Read the model definition and answer for the solid it produces. Units are mm, in the model's axes. A direction names the side the tool comes from. Coordinates: 2 decimals unless noted, no trailing zeros. Loops run counter-clockwise (first coordinate to the right, second up) from the corner with the lowest first, then second, coordinate; pieces in that order, holes last. Notation, with made-up numbers: (-2.5, 24) - (47.5, 24) arc R36 ccw to (47.5, 60) - close; hole circle Ø1 at (-9.5, 36.25). An arc over 180 degrees is marked (long way). One line per item, written item: value. Start each with the question number.
from build123d import *
from build123d.topology import SkipClean

# Parameters (mm, degrees)
SKETCH_1_R               = 27.5
EXTRUDE_1_DEPTH          = 4.5
SKETCH_2_R               = 9.75
EXTRUDE_2_DEPTH          = 30.8
CUT_EXTRUDE_1_DEPTH      = 28
SKETCH_5_R               = 10
EXTRUDE_3_DEPTH          = 7
SKETCH_6_R               = 8.5
EXTRUDE_4_DEPTH          = 8
SKETCH_11_R              = 2.5
CUT_EXTRUDE_3_DEPTH      = 50.609878049
PATTERN_CIRCULAR_1_COUNT = 6
SKETCH_12_R              = 13.008113322
CUT_EXTRUDE_4_DEPTH      = 25.8
CHAMFER_2_SIZE           = 1
SKETCH_13_W              = 0.4
SKETCH_13_H              = 1.1
CHAMFER_3_SIZE           = 0.5
CUT_EXTRUDE_5_DEPTH      = 46.964660338
SKETCH_15_R              = 1.6
CUT_EXTRUDE_6_DEPTH      = 25
HOLE_WIZARD_M3_1_D       = 2.5
SKETCH_18_R              = 27.5
CUT_EXTRUDE_7_DEPTH      = 44.505746792
PATTERN_CIRCULAR_2_COUNT = 3
PATTERN_CIRCULAR_2_ANGLE = 240
SKETCH_19_R              = 5
CUT_EXTRUDE_8_DEPTH      = 1


with BuildPart() as part:
    # 草图1 → 凸台-拉伸1 (new body)
    with BuildSketch(Plane(origin=(0, 0, 0), x_dir=(1, 0, 0), z_dir=(0, 1, 0))):
        with Locations(Location((0, 0, 0), (0, 0, 270))):
            Circle(SKETCH_1_R)
    extrude(amount=EXTRUDE_1_DEPTH)

    # 草图2 → 凸台-拉伸2 (add)
    with BuildSketch(Plane(origin=(0, 4.5, 0), x_dir=(1, 0, 0), z_dir=(0, 1, 0))):
        with Locations(Location((0, 0, 0), (0, 0, 90))):
            Circle(SKETCH_2_R)
    extrude(amount=EXTRUDE_2_DEPTH)

    # 草图4 → 切除-拉伸1 (cut)
    with BuildSketch(Plane(origin=(0, 35.3, 0), x_dir=(1, 0, 0), z_dir=(0, 1, 0))):
        with BuildLine():
            Line((-4, 3), (-4, -3))
            ThreePointArc((-4, -3), (5, 0), (-4, 3))
        make_face()
    extrude(amount=-CUT_EXTRUDE_1_DEPTH, mode=Mode.SUBTRACT)

    # 草图5 → 凸台-拉伸3 (add)
    with BuildSketch(Plane.XZ):
        with Locations(Location((0, 0, 0), (0, 0, 90))):
            Circle(SKETCH_5_R)
    extrude(amount=EXTRUDE_3_DEPTH)

    # 草图6 → 凸台-拉伸4 (add)
    with BuildSketch(Plane.XZ.offset(7)):
        with Locations(Location((0, 0, 0), (0, 0, 270))):
            Circle(SKETCH_6_R)
    extrude(amount=EXTRUDE_4_DEPTH)

    # 草图11 → 切除-拉伸3 (cut, through all)
    with BuildSketch(Plane(origin=(0, 4.5, 0), x_dir=(1, 0, 0), z_dir=(0, 1, 0))):
        with Locations(Location((-22.5, 0, 0), (0, 0, 270))):
            Circle(SKETCH_11_R)
    cut_extrude_3 = extrude(amount=-CUT_EXTRUDE_3_DEPTH, mode=Mode.SUBTRACT)

    # 阵列(圆周)1: 切除-拉伸3 ×6 about axis
    pattern_circular_1_axis = Axis((0, 0, 0), (0, 1, 0))
    for i in range(1, PATTERN_CIRCULAR_1_COUNT):
        add(cut_extrude_3.rotate(pattern_circular_1_axis, i * 360 / PATTERN_CIRCULAR_1_COUNT), mode=Mode.SUBTRACT)

    # 草图12 → 切除-拉伸4 (cut)
    with BuildSketch(Plane(origin=(0, 35.3, 0), x_dir=(1, 0, 0), z_dir=(0, 1, 0))):
        Circle(SKETCH_12_R)
    extrude(amount=-CUT_EXTRUDE_4_DEPTH, mode=Mode.SUBTRACT)

    # 倒角2
    chamfer_2_edges = [part.edges().sort_by_distance(p)[0] for p in [
        (0, 9.5, 9.75),
    ]]
    chamfer(chamfer_2_edges, length=CHAMFER_2_SIZE)

    # 草图13 → 切除-旋转1 (revolve, cut)
    with BuildSketch(Plane.XY, mode=Mode.PRIVATE) as cut_revolve_1_sk:
        with Locations((-8.3, -12.45)):
            Rectangle(SKETCH_13_W, SKETCH_13_H)
    revolve(cut_revolve_1_sk.sketch.rotate(Axis((0, 20.99290486, 0), (0, -1, 0)), 270), axis=Axis((0, 20.99290486, 0), (0, -1, 0)), mode=Mode.SUBTRACT)

    # 倒角3
    chamfer_3_edges = [part.edges().sort_by_distance(p)[0] for p in [
        (0, -15, 8.5),
    ]]
    chamfer(chamfer_3_edges, length=CHAMFER_3_SIZE)

    # 草图14 → 切除-拉伸5 (cut, through all)
    with BuildSketch(Plane.XZ.offset(15)):
        with BuildLine():
            Line((-4, -3), (-4, 3))
            ThreePointArc((-4, 3), (5, 0), (-4, -3))
        make_face()
    extrude(amount=-CUT_EXTRUDE_5_DEPTH, mode=Mode.SUBTRACT)

    # 草图15 → 切除-拉伸6 (cut)
    with BuildSketch(Plane(origin=(0, 0, 0), x_dir=(0, 0, -1), z_dir=(1, 0, 0))):
        with Locations(Location((0, -4, 0), (0, 0, 180))):
            Circle(SKETCH_15_R)
    extrude(amount=CUT_EXTRUDE_6_DEPTH, mode=Mode.SUBTRACT)

    # M3 螺纹孔1 (through all)
    with Locations(Plane(origin=(-4, 0, 0), x_dir=(0, 0, -1), z_dir=(1, 0, 0))):
        with Locations((0, -4)):
            Hole(HOLE_WIZARD_M3_1_D / 2)

    # 草图18 → 切除-拉伸7 (cut, through all)
    with BuildSketch(Plane(origin=(0, 4.5, 0), x_dir=(1, 0, 0), z_dir=(0, 1, 0))):
        with Locations((42, 0)):
            Circle(SKETCH_18_R)
    cut_extrude_7 = extrude(amount=-CUT_EXTRUDE_7_DEPTH, mode=Mode.SUBTRACT)

    # 阵列(圆周)2: 切除-拉伸7 ×3 about axis
    pattern_circular_2_axis = Axis((0, 0, 0), (0, 1, 0))
    for i in range(1, PATTERN_CIRCULAR_2_COUNT):
        add(cut_extrude_7.rotate(pattern_circular_2_axis, i * PATTERN_CIRCULAR_2_ANGLE / (PATTERN_CIRCULAR_2_COUNT - 1)), mode=Mode.SUBTRACT)

    # 倒角4
    # the kernel refuses this chamfer: 1.21981355, 1 mm, written as the material it takes off along each edge
    with BuildSketch(Plane(origin=(21, 7.559330204, 17.755280905), x_dir=(-0.6313868632849613, 0, -0.7754680063491838), z_dir=(0, -1, 0)), Plane(origin=(4.876524315, 7.559330204, -27.064173932), x_dir=(-0.3558815616779696, 0, 0.9345310663951465), z_dir=(0, -1, 0)), Plane(origin=(-25.876524315, 7.559330204, 9.308893027), x_dir=(0.9872684249629431, 0, -0.15906306004597578), z_dir=(0, -1, 0))) as chamfer_4_piece_1:
        with BuildLine():
            Line((1.019056312, 0), (-0.193408604, -1.168344991))
            ThreePointArc((-0.193408604, -1.168344991), (-0.106182465, -0.602433867), (0, 0))
            ThreePointArc((0, 0), (0.527109428, -0.00471513), (1.019056312, 0))
        make_face()
    extrude(amount=10.618660408, mode=Mode.SUBTRACT)
    with BuildSketch(Plane(origin=(21, 7.559330204, -17.755280905), x_dir=(-0.6313868632849639, 0, 0.7754680063491817), z_dir=(0, -1, 0))) as chamfer_4_piece_2:
        with BuildLine():
            Line((1.019056312, 0), (-0.193408604, 1.168344991))
            ThreePointArc((-0.193408604, 1.168344991), (-0.106182465, 0.602433867), (0, 0))
            ThreePointArc((0, 0), (0.527109428, 0.00471513), (1.019056312, 0))
        make_face()
    extrude(amount=10.618660408, mode=Mode.SUBTRACT)
    with BuildSketch(Plane(origin=(-25.876524315, 7.559330204, -9.308893027), x_dir=(-0.31816612737533284, 0, 0.9480349758268328), z_dir=(0, -1, 0)), Plane(origin=(4.876524315, 7.559330204, 27.064173932), x_dir=(0.9801054364298685, 0, -0.1984775389826691), z_dir=(0, -1, 0))) as chamfer_4_piece_3:
        with BuildLine():
            Line((1.18424529, 0), (-0.166430267, -1.005373928))
            ThreePointArc((-0.166430267, -1.005373928), (-0.08143465, -0.520802246), (0, 0))
            ThreePointArc((0, 0), (0.611686784, 0.006368493), (1.18424529, 0))
        make_face()
    extrude(amount=10.618660408, mode=Mode.SUBTRACT)

    # 草图19 → 切除-拉伸8 (cut)
    with SkipClean():  # the faces are left unmerged after this step: merging them gives an invalid solid
        with BuildSketch(Plane.XZ.offset(15)):
            with Locations(Location((0, 0, 0), (0, 0, 143.130102354))):
                Circle(SKETCH_19_R)
        extrude(amount=-CUT_EXTRUDE_8_DEPTH, mode=Mode.SUBTRACT)


solid = part.part
1) Section D-D, the plane z = 0 is taken. State how many separate pieces and enclosed holes the cut face has, and give its area (3 significant figures).
2) Section B-B, the plane z = 20 is taken. Determine the outline of the cut face in (x, y).
3) Determine the mould class of faces 1 (the cylindrical face through (-7.04, -5.22, -0.27)), 2 (the flat face through (-9, 0, 6)), 3 (the cylindrical face through (9.76, -3.45, -2.17)) for opening direction Z: released by +Z, released by -Z, zero draft, split by the parting line, or undercut.
4) Section C-C, the plane y = -4 is taken. Determine the outline of the cut face in (x, z), and give its area (3 significant figures).
5) Flat-ended cylindrical pins translate along their axes: P1, Ø4, axis at x = 11.25, z = 19.49, coming from the +Y side; P2, Ø3, axis at x = 11, z = -5, coming from the +Y side; P3, Ø1.5, axis at x = -12, z = -10.5, coming from the -Y side; P4, Ø1.5, axis at y = -7.5, z = -4, coming from the +X side. Find the tip coordinate at first contact, or state that the pin passes through.
6) Section A-A, the plane x = -22.5 is taken. Determine the outline of the cut face in (y, z), and give its area (3 significant figures).
7) Straight lines are drawn through the part: L1, parallel to X at y = 3.25, z = 0; L2, parallel to Z at x = 9, y = 0.5; L3, parallel to Z at x = 10, y = 0.25. For each, find the intervals that lie inside material, in ascending order.
8) For faces 4 (the cylindrical face through (8.428, -9.416, 1.107)), 5 (the cylindrical face through (-9.667, 6.472, 1.269)), 6 (the cylindrical face through (7.33, -3.39, 1.48)), 7 (the flat face through (5.286, 2.281, 26.476)), determine the directions among +Z, -Z, +X, -X, +Y, -Y from which every point of the face is accessible in a straight line to the end or side of a thin tool.
Answer below:
1. separate pieces: 5
1. enclosed holes: 0
1. area: 285 mm2
2. outline: (1.09, 0) - (8.8, 0) - (8.8, 4.5) - (1.09, 4.5) - close; (13.7, 0) - (18.87, 0) - (18.87, 4.5) - (13.7, 4.5) - close
3. face 1: undercut
3. face 2: zero draft
3. face 3: split by the parting line
4. outline: (-9.92, -1.25) arc R10 ccw to (9.87, -1.6) - (4.74, -1.6) arc R5 cw to (-4, -3) - (-4, -1.25) - close; (-9.92, 1.25) - (-4, 1.25) - (-4, 3) arc R5 cw to (4.74, 1.6) - (9.87, 1.6) arc R10 ccw to start
4. area: 209 mm2
5. P1: through
5. P2: y = 4.5
5. P3: y = 0
5. P4: x = 9.39
6. outline: (0, -8.91) - (4.5, -8.91) - (4.5, -2.5) - (0, -2.5) - close; (0, 2.5) - (4.5, 2.5) - (4.5, 8.91) - (0, 8.91) - close
6. area: 57.7 mm2
7. L1: -27.5 to -25, -20 to -4, 5 to 14.5
7. L2: -25.99 to -20.58, -18.4 to 18.4, 20.58 to 25.99
7. L3: -25.62 to -21.65, -17.32 to 17.32, 21.65 to 25.62
8. face 4: -Y
8. face 5: +Y
8. face 6: +X
8. face 7: +Z, -X, +Y, -Y
